```python
from build123d import *

# Parameters (mm, degrees)
SKETCH1_W                         = 125
SKETCH1_H                         = 120
TOP_BASE_DEPTH                    = 9
SKETCH5_R                         = 14.15
DRIVE_GEAR_HOLE_DEPTH             = 6
SKETCH28_R                        = 15.15
TWO_STAGE_GEAR_HOLE_DEPTH         = 174.51080658
SKETCH8_R                         = 18.5
XL320_FINGER_KNUCKLE_MOUNT_DEPTH  = 174.51080658
SKETCH26_R                        = 1
STRING_HOLES_DEPTH                = 174.51080658
XL320_MOUNT_HOLES_R               = 2.25
XL320_MOUNT_HOLES_M4_DEPTH        = 174.51080658
AX12_MOUNT_HOLES_R                = 2.25
AX12_MOUNT_HOLES_M4_DEPTH         = 174.51080658
NUTS_M4_DEPTH                     = 5
SKETCH34_R                        = 15
HOLES_FOR_M4_IN_FINGER_GEAR_DEPTH = 2
SKETCH31_W                        = 38
SKETCH31_H                        = 15
BOSS_EXTRUDE1_DEPTH               = 10
SKETCH32_R                        = 15.25
CUT_EXTRUDE5_DEPTH                = 5
SKETCH33_R                        = 1
CUT_EXTRUDE6_DEPTH                = 2.5
FILLET2_R                         = 10
CUT_EXTRUDE8_DEPTH                = 174.565549577
FILLET4_R                         = 10
SKETCH37_R                        = 3.25
CONNECT_HOLES_M6_DEPTH            = 10
SKETCH41_R                        = 2
CONNECT_TO_HOUSE_M4_DEPTH         = 174.565549577
SKETCH42_W                        = 3
SKETCH42_H                        = 9
HOUSING_FITS_DEPTH                = 5
HOUSING_FITS_DRAFT                = 5
HOUSING_FITS_PROFILE_2_DEPTH      = 5
HOUSING_FITS_PROFILE_2_DRAFT      = 5
HOUSING_FITS_PROFILE_3_DEPTH      = 5
HOUSING_FITS_PROFILE_3_DRAFT      = 5
HOUSING_FITS_PROFILE_4_DEPTH      = 5
HOUSING_FITS_PROFILE_4_DRAFT      = 5
SKETCH43_R                        = 1
M2_SHAFT_HOLE_DEPTH               = 2
SKETCH44_R                        = 1.05
CUT_EXTRUDE9_DEPTH                = 5
SKETCH45_R                        = 1.05
CUT_EXTRUDE10_DEPTH               = 2.5


with BuildPart() as part:
    # Sketch1 → Top_Base (new body)
    with BuildSketch(Plane(origin=(0, 0, 0), x_dir=(1, 0, 0), z_dir=(0, 1, 0))):
        with BuildLine():
            ThreePointArc((0, 120), (-13.654246239, 60), (0, 0))
            Line((0, 0), (0, 120))
        make_face()
        with Locations((62.5, 60)):
            Rectangle(SKETCH1_W, SKETCH1_H)
    extrude(amount=TOP_BASE_DEPTH)

    # Sketch5 → Drive_Gear_Hole (cut)
    with BuildSketch(Plane(origin=(0, 9, 0), x_dir=(1, 0, 0), z_dir=(0, 1, 0))):
        with Locations(Location((23.75, 73.41386581, 0), (0, 0, 270))):
            Circle(SKETCH5_R)
    extrude(amount=-DRIVE_GEAR_HOLE_DEPTH, mode=Mode.SUBTRACT)

    # Sketch28 → Two_Stage_Gear_Hole (cut, through all)
    with BuildSketch(Plane(origin=(0, 9, 0), x_dir=(1, 0, 0), z_dir=(0, 1, 0))):
        with Locations(Location((39.169567191, 51.25, 0), (0, 0, 270))):
            Circle(SKETCH28_R)
    extrude(amount=-TWO_STAGE_GEAR_HOLE_DEPTH, mode=Mode.SUBTRACT)

    # Sketch8 → XL320_Finger_Knuckle_Mount (cut, through all)
    with BuildSketch(Plane(origin=(0, 9, 0), x_dir=(1, 0, 0), z_dir=(0, 1, 0))):
        with Locations(Location((104.5, 60, 0), (0, 0, 270))):
            Circle(SKETCH8_R)
    extrude(amount=-XL320_FINGER_KNUCKLE_MOUNT_DEPTH, mode=Mode.SUBTRACT)

    # Sketch26 → String_Holes (cut, through all)
    with BuildSketch(Plane.XZ.offset(-9)):
        with Locations(Location((26, -30, 0), (0, 0, 270))):
            Circle(SKETCH26_R)
        with Locations(Location((26, -90, 0), (0, 0, 90))):
            Circle(SKETCH26_R)
    extrude(amount=STRING_HOLES_DEPTH, mode=Mode.SUBTRACT)

    # XL320_Mount_Holes → XL320_Mount_Holes_(M4) (cut, through all)
    with BuildSketch(Plane(origin=(0, 9, 0), x_dir=(1, 0, 0), z_dir=(0, 1, 0))):
        with Locations(Location((110.5, 36, 0), (0, 0, 270))):
            Circle(XL320_MOUNT_HOLES_R)
        with Locations(Location((98.5, 36, 0), (0, 0, 270))):
            Circle(XL320_MOUNT_HOLES_R)
        with Locations(Location((-0.25, 79.41386581, 0), (0, 0, 270))):
            Circle(XL320_MOUNT_HOLES_R)
        with Locations(Location((-0.25, 67.41386581, 0), (0, 0, 270))):
            Circle(XL320_MOUNT_HOLES_R)
    extrude(amount=-XL320_MOUNT_HOLES_M4_DEPTH, mode=Mode.SUBTRACT)

    # AX12_Mount_Holes → AX12_Mount_Holes_(M4) (cut, through all)
    with BuildSketch(Plane(origin=(0, 9, 0), x_dir=(1, 0, 0), z_dir=(0, 1, 0))):
        with Locations(Location((72.25, 112.25, 0), (0, 0, 270))):
            Circle(AX12_MOUNT_HOLES_R)
        with Locations(Location((63.25, 80.25, 0), (0, 0, 270))):
            Circle(AX12_MOUNT_HOLES_R)
        with Locations(Location((73.25, 100, 0), (0, 0, 270))):
            Circle(AX12_MOUNT_HOLES_R)
        with Locations(Location((93.75, 109, 0), (0, 0, 270))):
            Circle(AX12_MOUNT_HOLES_R)
        with Locations(Location((63.25, 39.75, 0), (0, 0, 270))):
            Circle(AX12_MOUNT_HOLES_R)
        with Locations(Location((72.25, 7.75, 0), (0, 0, 270))):
            Circle(AX12_MOUNT_HOLES_R)
    extrude(amount=-AX12_MOUNT_HOLES_M4_DEPTH, mode=Mode.SUBTRACT)

    # Sketch27 → Nuts_(M4) (cut)
    with BuildSketch(Plane.XZ):
        Polygon((110.5, -31.958548116), (107, -33.979274058), (107, -38.020725942), (110.5, -40.041451884), (114, -38.020725942), (114, -33.979274058), align=None)
        Polygon((98.5, -31.958548116), (95, -33.979274058), (95, -38.020725942), (98.5, -40.041451884), (102, -38.020725942), (102, -33.979274058), align=None)
        Polygon((3.25, -65.393139868), (-0.25, -63.372413926), (-3.75, -65.393139868), (-3.75, -69.434591752), (-0.25, -71.455317694), (3.25, -69.434591752), align=None)
        Polygon((-3.75, -77.393139868), (-3.75, -81.434591752), (-0.25, -83.455317694), (3.25, -81.434591752), (3.25, -77.393139868), (-0.25, -75.372413926), align=None)
    extrude(amount=-NUTS_M4_DEPTH, mode=Mode.SUBTRACT)

    # Sketch34 → Holes_For_M4_In_Finger_Gear (cut)
    with BuildSketch(Plane.XZ):
        with Locations((26, -30)):
            Circle(SKETCH34_R)
        with Locations(Location((26, -90, 0), (0, 0, 270))):
            Circle(SKETCH34_R)
    extrude(amount=-HOLES_FOR_M4_IN_FINGER_GEAR_DEPTH, mode=Mode.SUBTRACT)

    # Sketch31 → Boss-Extrude1 (add)
    with BuildSketch(Plane(origin=(0, 9, 0), x_dir=(1, 0, 0), z_dir=(0, 1, 0))):
        with Locations((39.169567191, 51.25)):
            Rectangle(SKETCH31_W, SKETCH31_H)
    extrude(amount=BOSS_EXTRUDE1_DEPTH)

    # Sketch32 → Cut-Extrude5 (cut)
    with BuildSketch(Plane.XZ.offset(-9)):
        with Locations((39.169567191, -51.25)):
            Circle(SKETCH32_R)
    extrude(amount=-CUT_EXTRUDE5_DEPTH, mode=Mode.SUBTRACT)

    # Sketch33 → Cut-Extrude6 (cut)
    with BuildSketch(Plane.XZ.offset(-14)):
        with Locations(Location((39.169567191, -51.25, 0), (0, 0, 270))):
            Circle(SKETCH33_R)
    extrude(amount=-CUT_EXTRUDE6_DEPTH, mode=Mode.SUBTRACT)

    # Fillet2
    fillet2_edges = [part.edges().sort_by_distance(p)[0] for p in [
        (58.169567191, 19, -51.25),
        (20.169567191, 19, -51.25),
    ]]
    fillet(fillet2_edges, radius=FILLET2_R - 0.0001)  # a hair under: the kernel refuses the full size

    # Sketch36 → Cut-Extrude8 (cut, through all)
    with BuildSketch(Plane(origin=(0, 9, 0), x_dir=(1, 0, 0), z_dir=(0, 1, 0))):
        Polygon((90, 120), (125, 100), (125, 120), align=None)
        Polygon((125, 0), (90, 0), (125, 20), align=None)
    extrude(amount=-CUT_EXTRUDE8_DEPTH, mode=Mode.SUBTRACT)

    # Fillet4
    fillet4_edges = [part.edges().sort_by_distance(p)[0] for p in [
        (90, 4.5, -120),
        (125, 4.5, -100),
        (125, 4.5, -20),
        (90, 4.5, 0),
        (0, 4.5, -120),
        (0, 4.5, 0),
    ]]
    fillet(fillet4_edges, radius=FILLET4_R)

    # Sketch37 → Connect_Holes_(M6) (cut)
    with BuildSketch(Plane(origin=(0, 9, 0), x_dir=(1, 0, 0), z_dir=(0, 1, 0))):
        with Locations(Location((4.459226107, 111.152938298, 0), (0, 0, 270))):
            Circle(SKETCH37_R)
        with Locations(Location((4.459226107, 8.847061702, 0), (0, 0, 270))):
            Circle(SKETCH37_R)
        with Locations(Location((91.344355629, 8.205555711, 0), (0, 0, 270))):
            Circle(SKETCH37_R)
    extrude(amount=-CONNECT_HOLES_M6_DEPTH, mode=Mode.SUBTRACT)

    # Sketch41 → Connect_To_House_(M4) (cut, through all)
    with BuildSketch(Plane(origin=(0, 9, 0), x_dir=(1, 0, 0), z_dir=(0, 1, 0))):
        with Locations(Location((65, 60, 0), (0, 0, 270))):
            Circle(SKETCH41_R)
    extrude(amount=-CONNECT_TO_HOUSE_M4_DEPTH, mode=Mode.SUBTRACT)


with BuildPart() as housing_fits_tool:
    # Sketch42 → Housing_Fits (with draft: the straight prism first)
    with BuildSketch(Plane(origin=(0, 9, 0), x_dir=(1, 0, 0), z_dir=(0, 1, 0))):
        with Locations((122.5, 30.5)):
            Rectangle(SKETCH42_W, SKETCH42_H)
    extrude(amount=HOUSING_FITS_DEPTH)
    # Housing_Fits: the draft: its side faces are tilted about the plane it starts from
    housing_fits_sides = [housing_fits_tool.faces().sort_by_distance(p)[0] for p in [
        (124, 11.5, -30.5),
        (122.5, 11.5, -35),
        (121, 11.5, -30.5),
        (122.5, 11.5, -26),
    ]]
    draft(housing_fits_sides, Plane(origin=(0, 9, 0), x_dir=(1, 0, 0), z_dir=(0, 1, 0)), HOUSING_FITS_DRAFT)


with BuildPart() as part_1:
    add(part.part)

    # Housing_Fits: add housing_fits_tool
    add(housing_fits_tool.part)


with BuildPart() as housing_fits_profile_2_tool:
    # Sketch42 → Housing_Fits profile 2 (with draft: the straight prism first)
    with BuildSketch(Plane(origin=(0, 9, 0), x_dir=(1, 0, 0), z_dir=(0, 1, 0))):
        Polygon((-9.533377338, 30.232888291), (-7.782151246, 21.404909633), (-4.349048435, 22.085942002), (-6.100274527, 30.91392066), align=None)
    extrude(amount=HOUSING_FITS_PROFILE_2_DEPTH)
    # Housing_Fits profile 2: the draft: its side faces are tilted about the plane it starts from
    housing_fits_profile_2_sides = [housing_fits_profile_2_tool.faces().sort_by_distance(p)[0] for p in [
        (-8.657764292, 11.5, -25.818898962),
        (-6.065599841, 11.5, -21.745425818),
        (-5.224661481, 11.5, -26.499931331),
        (-7.816825933, 11.5, -30.573404475),
    ]]
    draft(housing_fits_profile_2_sides, Plane(origin=(0, 9, 0), x_dir=(1, 0, 0), z_dir=(0, 1, 0)), HOUSING_FITS_PROFILE_2_DRAFT)


with BuildPart() as part_2:
    add(part_1.part)

    # Housing_Fits profile 2: add housing_fits_profile_2_tool
    add(housing_fits_profile_2_tool.part)


with BuildPart() as housing_fits_profile_3_tool:
    # Sketch42 → Housing_Fits profile 3 (with draft: the straight prism first)
    with BuildSketch(Plane(origin=(0, 9, 0), x_dir=(1, 0, 0), z_dir=(0, 1, 0))):
        Polygon((-4.349048435, 97.914057998), (-7.782151246, 98.595090367), (-9.533377338, 89.767111709), (-6.100274527, 89.08607934), align=None)
    extrude(amount=HOUSING_FITS_PROFILE_3_DEPTH)
    # Housing_Fits profile 3: the draft: its side faces are tilted about the plane it starts from
    housing_fits_profile_3_sides = [housing_fits_profile_3_tool.faces().sort_by_distance(p)[0] for p in [
        (-6.065599841, 11.5, -98.254574182),
        (-8.657764292, 11.5, -94.181101038),
        (-7.816825933, 11.5, -89.426595525),
        (-5.224661481, 11.5, -93.500068669),
    ]]
    draft(housing_fits_profile_3_sides, Plane(origin=(0, 9, 0), x_dir=(1, 0, 0), z_dir=(0, 1, 0)), HOUSING_FITS_PROFILE_3_DRAFT)


with BuildPart() as part_3:
    add(part_2.part)

    # Housing_Fits profile 3: add housing_fits_profile_3_tool
    add(housing_fits_profile_3_tool.part)


with BuildPart() as housing_fits_profile_4_tool:
    # Sketch42 → Housing_Fits profile 4 (with draft: the straight prism first)
    with BuildSketch(Plane(origin=(0, 9, 0), x_dir=(1, 0, 0), z_dir=(0, 1, 0))):
        with Locations((122.5, 89.5)):
            Rectangle(SKETCH42_W, SKETCH42_H)
    extrude(amount=HOUSING_FITS_PROFILE_4_DEPTH)
    # Housing_Fits profile 4: the draft: its side faces are tilted about the plane it starts from
    housing_fits_profile_4_sides = [housing_fits_profile_4_tool.faces().sort_by_distance(p)[0] for p in [
        (122.5, 11.5, -94),
        (121, 11.5, -89.5),
        (122.5, 11.5, -85),
        (124, 11.5, -89.5),
    ]]
    draft(housing_fits_profile_4_sides, Plane(origin=(0, 9, 0), x_dir=(1, 0, 0), z_dir=(0, 1, 0)), HOUSING_FITS_PROFILE_4_DRAFT)


with BuildPart() as part_4:
    add(part_3.part)

    # Housing_Fits profile 4: add housing_fits_profile_4_tool
    add(housing_fits_profile_4_tool.part)

    # Sketch43 → M2_Shaft_Hole (cut)
    with BuildSketch(Plane.XZ):
        with Locations(Location((39.169567191, -68.75, 0), (0, 0, 270))):
            Circle(SKETCH43_R)
    extrude(amount=-M2_SHAFT_HOLE_DEPTH, mode=Mode.SUBTRACT)

    # Sketch44 → Cut-Extrude9 (cut)
    with BuildSketch(Plane(origin=(0, 9, 0), x_dir=(1, 0, 0), z_dir=(0, 1, 0))):
        with Locations(Location((-2.75, 46.75, 0), (0, 0, 270))):
            Circle(SKETCH44_R)
        with Locations(Location((40.25, 70.75, 0), (0, 0, 270))):
            Circle(SKETCH44_R)
        with Locations(Location((57.75, 70.75, 0), (0, 0, 270))):
            Circle(SKETCH44_R)
    extrude(amount=-CUT_EXTRUDE9_DEPTH, mode=Mode.SUBTRACT)

    # Sketch45 → Cut-Extrude10 (cut)
    with BuildSketch(Plane(origin=(0, 19, 0), x_dir=(1, 0, 0), z_dir=(0, 1, 0))):
        with Locations(Location((37.25, 46.75, 0), (0, 0, 270))):
            Circle(SKETCH45_R)
    extrude(amount=-CUT_EXTRUDE10_DEPTH, mode=Mode.SUBTRACT)


solid = part_4.part
```
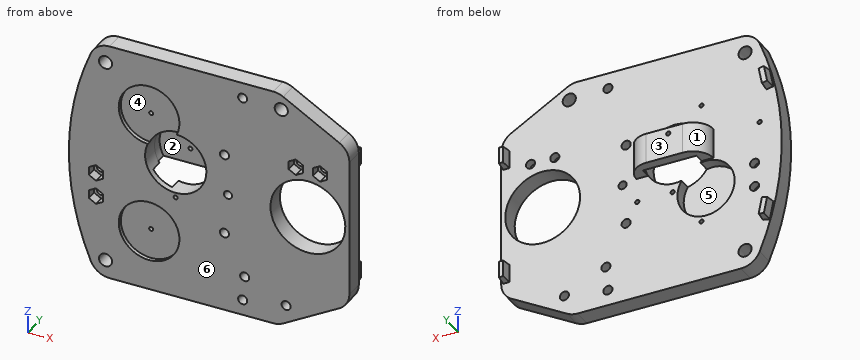
The listing builds one solid part. Answer for the finished solid, in the listing's coordinates (mm). Face numbers are marked on the shaded views. A direction names the side the tool comes from. Coordinates: 2 decimals unless noted, no trailing zeros. Loops run counter-clockwise (first coordinate to the right, second up) from the corner with the lowest first, then second, coordinate; pieces in that order, holes last. Notation, with made-up numbers: (87, -16.75) - (117, -16.75) arc R11 cw to (117, 0.25) - close; hole circle Ø6 at (85.5, 12). An arc over 180 degrees is marked (long way). Use a Markdown table: item, result. Add a question column.
1) The part is cut by section A-A, the plane y = 10.75. Give the vertices of the cut face in (x, z).
2) Given pin 1 (2.5 mm diameter, centred on x = 39.17, z = -51.25, fed in from -Y); pin 2 (3.5 mm diameter, centred on x = -7.5, z = -27, fed in from +Y); pin 3 (5 mm diameter, centred on x = 74, z = -67, fed in from +Y), each flat-ended and moving along its own axis, determine where each tip first touches the part or whether it passes through.
3) The part is cut by section B-B, the plane x = 104.5. Give the vertices of the cut face in (y, z).
4) Find the intervals of material crossed by line 1 (X direction, y = 8.15, z = -36); line 2 (Z direction, x = 54.5, y = 16.25); line 3 (Z direction, x = 92, y = 1.5), in increasing order.
5) For the marked faces 4, 5 and 6, determine the directions among +Z, -Z, +X, -X, +Y, -Y from which every point of the face is accessible in a straight line to the end or side of a thin tool.
6) The mould has two halves that part along X. Classify the marked faces 1, 2 and 3: released by +X, released by -X, zero draft, split by the parting line, or undercut.
7) The part is cut by section C-C, the plane x = 80. Give the vertices of the cut face in (y, z), and give its area (3 significant figures).
Here are the results:
| question | item | result |
|---|---|---|
| 1 | outline | (-9.35, -89.89) - (-7.66, -98.42) - (-4.53, -97.79) - (-6.22, -89.27) - close; (-9.35, -30.11) - (-6.22, -30.73) - (-4.53, -22.21) - (-7.66, -21.58) - close; (20.32, -58.75) - (25.89, -58.75) arc R15.25 cw to (25.89, -43.75) - (20.32, -43.75) - close; (52.45, -58.75) - (58.02, -58.75) - (58.02, -43.75) - (52.45, -43.75) arc R15.25 cw to start; (121.15, -93.85) - (123.85, -93.85) - (123.85, -85.15) - (121.15, -85.15) - close; (121.15, -34.85) - (123.85, -34.85) - (123.85, -26.15) - (121.15, -26.15) - close |
| 2 | pin 1 | stops at y = 14 |
| 2 | pin 2 | stops at y = 14 |
| 2 | pin 3 | stops at y = 9 |
| 3 | outline | (0, -111.71) - (9, -111.71) - (9, -78.5) - (0, -78.5) - close; (0, -41.5) - (9, -41.5) - (9, -8.29) - (0, -8.29) - close |
| 4 | line 1 | x = -11.56 to 96.25, 100.75 to 108.25, 112.75 to 125 |
| 4 | line 2 | z = -58.75 to -43.75 |
| 4 | line 3 | z = -118.85 to -110.41, -107.59 to -73.64, -46.36 to -11.39, -5.02 to -1.15 |
| 5 | face 4 | -Y |
| 5 | face 5 | +Y |
| 5 | face 6 | +Z, -Z, +X, -X, -Y |
| 6 | face 1 | released by -X |
| 6 | face 2 | undercut |
| 6 | face 3 | zero draft |
| 7 | outline | (0, -120) - (9, -120) - (9, 0) - (0, 0) - close |
| 7 | area | 1,080 mm^2 |
